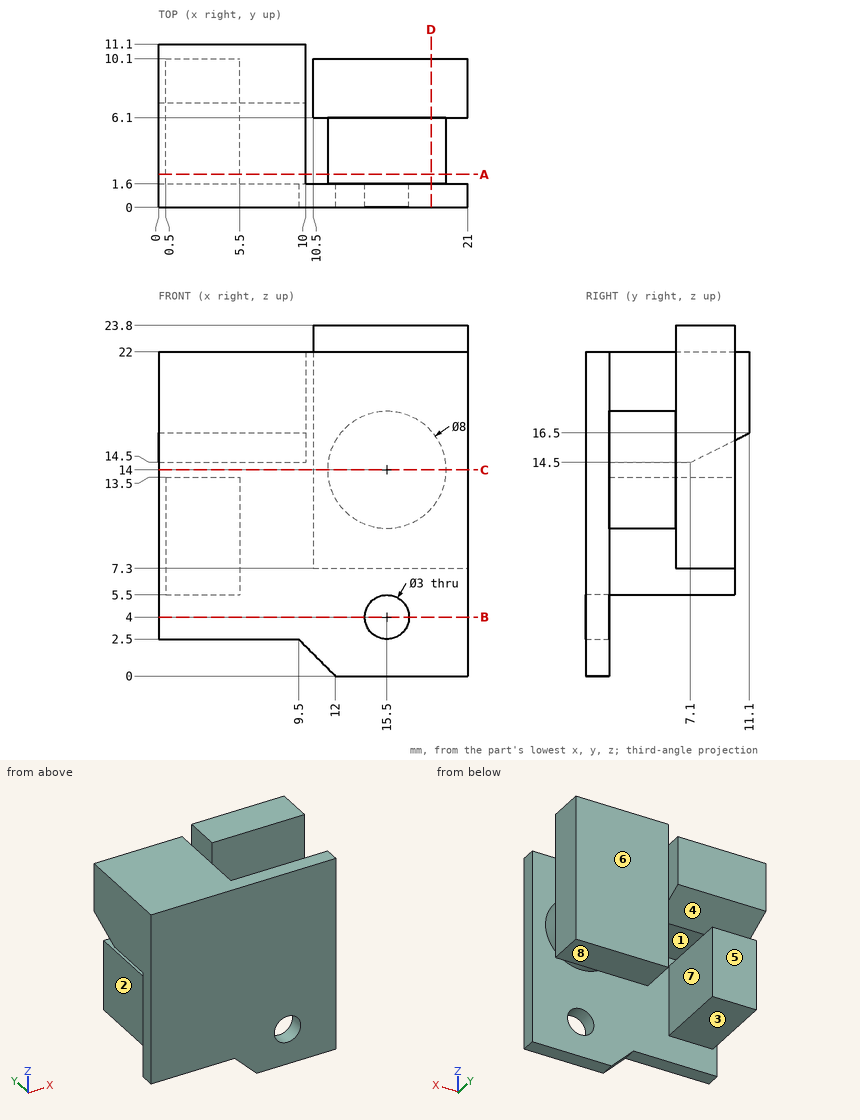
The drawing under review shows one solid part. Ordinate dimensions are in mm from its lowest x, y, z. A direction names the side the tool comes from. Give positions to 0.01 mm unless a question says otherwise; leave off trailing zeros. Loops run counter-clockwise (first coordinate to the right, second up) from the corner with the lowest first, then second, coordinate; pieces in that order, holes last. Notation, with made-up numbers: M 11,-40 L 21,-40 A15 ccw 21,-21 Z; hole C 56.5,27.25 d7. An arc over 180 degrees is marked long. One line per item, written item: value. Start each with the question number.
Q1. Machinability: for the marked faces 5, 6, 7 and 8, which of the approach directions +Z, -Z, +X, -X, +Y, -Y give a long, thin tool a straight path to every point of the face, cutting with its end or side? Answer none if there is none.
Q2. Add section C-C (z = 14). Give the boundary of the cut face in (x, y).
Q3. Add section A-A (y = 2.25). Give the boundary of the cut face in (x, z), and give its area (3 significant figures).
Q4. Clearance check with flat-ended pins moving along their axes: pin 1 Ø1 at (x, y) = (13.5, 6.5) entering from -Z; pin 2 Ø10 at (x, z) = (10.5, 19.5) entering from -Y; pin 3 Ø3 at (x, y) = (4.5, 3) entering from -Z; pin 4 Ø3 at (x, z) = (16, 15) entering from +Y. State where each tip first meets the part, or that it passes through.
Q5. Add section B-B (z = 4). Give the boundary of the cut face in (x, y).
Q6. Add section D-D (x = 18.5). Give the boundary of the cut face in (y, z).
Q7. Draft analysis for pull direction Z (two halves, no side actions). For the marked faces 1, 2, 3 and 4, state which applies: released by +Z, released by -Z, zero draft, split by the parting line, or undercut.
Q8. For L1, parallel to Z at x = 3.75, y = 7; L2, parallel to X at y = 7.75, z = 20; L3, parallel to X at y = 1.1, z = 4, list the stretches that pass through material, from the lowest coordinate up.
Reply:
1. face 5: -Z, +X, -X, +Y
1. face 6: +Z, -Z, +X, +Y
1. face 7: -Z, +Y
1. face 8: -Z, +X, +Y
2. outline: M 0,0 L 21,0 L 21,1.6 L 19.5,1.6 L 19.5,6.1 L 21,6.1 L 21,10.1 L 10.5,10.1 L 10.5,6.1 L 11.5,6.1 L 11.5,1.6 L 0,1.6 Z
3. outline: M 0,14.5 L 10,14.5 L 10,22 L 0,22 Z; M 0.5,5.5 L 5.5,5.5 L 5.5,13.5 L 0.5,13.5 Z; C 15.5,14 d8
3. area: 165 mm²
4. pin 1: z = 7.3
4. pin 2: y = 0
4. pin 3: z = 2.5
4. pin 4: y = 10.1
5. outline: M 0,0 L 14,0 L 14,1.6 L 0,1.6 Z; M 17,0 L 21,0 L 21,1.6 L 17,1.6 Z
6. outline: M 0,0 L 1.6,0 L 1.6,11.35 L 6.1,11.35 L 6.1,7.3 L 10.1,7.3 L 10.1,23.8 L 6.1,23.8 L 6.1,16.65 L 1.6,16.65 L 1.6,22 L 0,22 Z
7. face 1: undercut
7. face 2: zero draft
7. face 3: released by -Z
7. face 4: undercut
8. L1: 5.5 to 13.5, 14.5 to 22
8. L2: 0 to 10, 10.5 to 21
8. L3: 0 to 14, 17 to 21
